from build123d import *

# Parameters (mm, degrees)
ESQUISSE1_R             = 0.76020263
BOSS_EXTRU_1_DEPTH      = 5
ESQUISSE2_W             = 30
ESQUISSE2_H             = 5
BOSS_EXTRU_2_DEPTH      = 20
ESQUISSE4_R             = 5
BOSS_EXTRU_3_DEPTH      = 15
ESQUISSE5_R             = 15
BOSS_EXTRU_4_DEPTH      = 50
ESQUISSE8_W             = 0.1
ESQUISSE8_H             = 0.1
ENL_V_MAT_EXTRU_1_DEPTH = 15
ESQUISSE7_R             = 5
BOSS_EXTRU_6_DEPTH      = 15


with BuildPart() as part:
    # Esquisse1 → Boss.-Extru.1 (new body)
    with BuildSketch(Plane.XY):
        with BuildLine():
            Line((-15, 35), (15, 35))
            Line((15, 35), (15, -34.999999772))
            ThreePointArc((15, -34.999999772), (1.14e-07, -49.999999886), (-15, -35))
            Line((-15, -35), (-15, 35))
        make_face()
        with Locations((0, -34.999999886)):
            Circle(ESQUISSE1_R, mode=Mode.SUBTRACT)
    extrude(amount=BOSS_EXTRU_1_DEPTH)

    # Esquisse2 → Boss.-Extru.2 (add)
    with BuildSketch(Plane(origin=(0, 0, 0), x_dir=(-1, 0, 0), z_dir=(0, 0, -1))):
        with Locations((0, 32.5)):
            Rectangle(ESQUISSE2_W, ESQUISSE2_H)
    extrude(amount=BOSS_EXTRU_2_DEPTH)

    # Esquisse4 → Boss.-Extru.3 (add)
    with BuildSketch(Plane.XY.offset(5)):
        with Locations((0, -34.999999886)):
            Circle(ESQUISSE4_R)
    extrude(amount=BOSS_EXTRU_3_DEPTH)

    # Esquisse5 → Boss.-Extru.4 (add)
    with BuildSketch(Plane(origin=(0, 0, 0), x_dir=(-1, 0, 0), z_dir=(0, 0, -1))):
        with Locations((0, -30)):
            Circle(ESQUISSE5_R)
    extrude(amount=BOSS_EXTRU_4_DEPTH)

    # Esquisse8 → Enlèv. mat.-Extru.1 (cut)
    with BuildSketch(Plane.XY.offset(20)):
        with Locations((0, -34.999999886)):
            Rectangle(ESQUISSE8_W, ESQUISSE8_H)
    extrude(amount=-ENL_V_MAT_EXTRU_1_DEPTH, mode=Mode.SUBTRACT)

    # Esquisse7 → Boss.-Extru.6 (add)
    with BuildSketch(Plane.XY.offset(20)):
        with Locations((0, -34.999999886)):
            Circle(ESQUISSE7_R)
    extrude(amount=BOSS_EXTRU_6_DEPTH)


solid = part.part
For this review, take the finished solid that the model builds, in its own axes (mm). A direction names the side the tool comes from. Coordinates: 2 decimals unless noted, no trailing zeros. Order: outer loops, then holes, each group sorted by start corner. A loop starts at its lowest first (then second) coordinate and runs counter-clockwise, first axis right, second up. Notation, with made-up numbers: (49, -21.75) -> (82, -21.75) arc R19 ccw to (82, 14.25) -> close; hole circle Ø1 at (87, 87). An arc over 180 degrees is marked (long way). Return JSON: item names as keys, results as strings.
1. We need section D-D on x = -2.5. Write out the cut boundary in (y, z).
Answer block:
{"outline": "(-49.79, 0) -> (-44.79, 0) -> (-44.79, -50) -> (-15.21, -50) -> (-15.21, 0) -> (30, 0) -> (30, -20) -> (35, -20) -> (35, 5) -> (-30.67, 5) -> (-30.67, 35) -> (-39.33, 35) -> (-39.33, 5) -> (-49.79, 5) -> close"}
2. Machinability: for faces 1 (the flat face through (0, 33, -20)), 2 (the flat face through (1, -46, 0)), 3 (the cylindrical face through (3.252, -44.643, -24.65)), 4 (the cylindrical face through (-1.08, -39.88, 19.79)), 5 (the flat face through (0, 30, -10)), which of the approach directions +Z, -Z, +X, -X, +Y, -Y give a long, thin tool a straight path to every point of the face, cutting with its end or side? Answer none if there is none.
Answer block:
{"face 1": "-Z, +X, -X, +Y", "face 2": "-Z, -Y", "face 3": "-Z", "face 4": "+Z", "face 5": "-Z, +X, -X"}
3. We need section B-B on z = 15.5. Write out the cut boundary in (x, y), and give its area (3 significant figures).
Answer block:
{"outline": "circle Ø10 at (0, -35); hole (-0.05, -35.05) -> (0.05, -35.05) -> (0.05, -34.95) -> (-0.05, -34.95) -> close", "area": "78.5 mm²"}
4. We need section A-A on z = -2.5. Write out the cut boundary in (x, y), and give its area (3 significant figures).
Answer block:
{"outline": "circle Ø30 at (0, -30); (-15, 30) -> (15, 30) -> (15, 35) -> (-15, 35) -> close", "area": "857 mm²"}
5. For pin 1 Ø1.5 at (x, y) = (-6.5, 33) entering from -Z; pin 2 Ø12 at (x, y) = (0, 24) entering from +Z; pin 3 Ø6 at (x, y) = (1, -8.5) entering from -Z, all flat-tipped, find the tip position at first contact; note any pin that passes through.
Answer block:
{"pin 1": "z = -20", "pin 2": "z = 5", "pin 3": "z = 0"}
6. For line 1 (Y direction, x = 0, z = 3.2); line 2 (Z direction, x = 0, y = 26); line 3 (Z direction, x = 1, y = -43), list the stretches that pass through material, from the lowest coordinate up. Write a range as from..to.
Answer block:
{"line 1": "-50..-35.76, -34.24..35", "line 2": "0..5", "line 3": "-50..5"}
